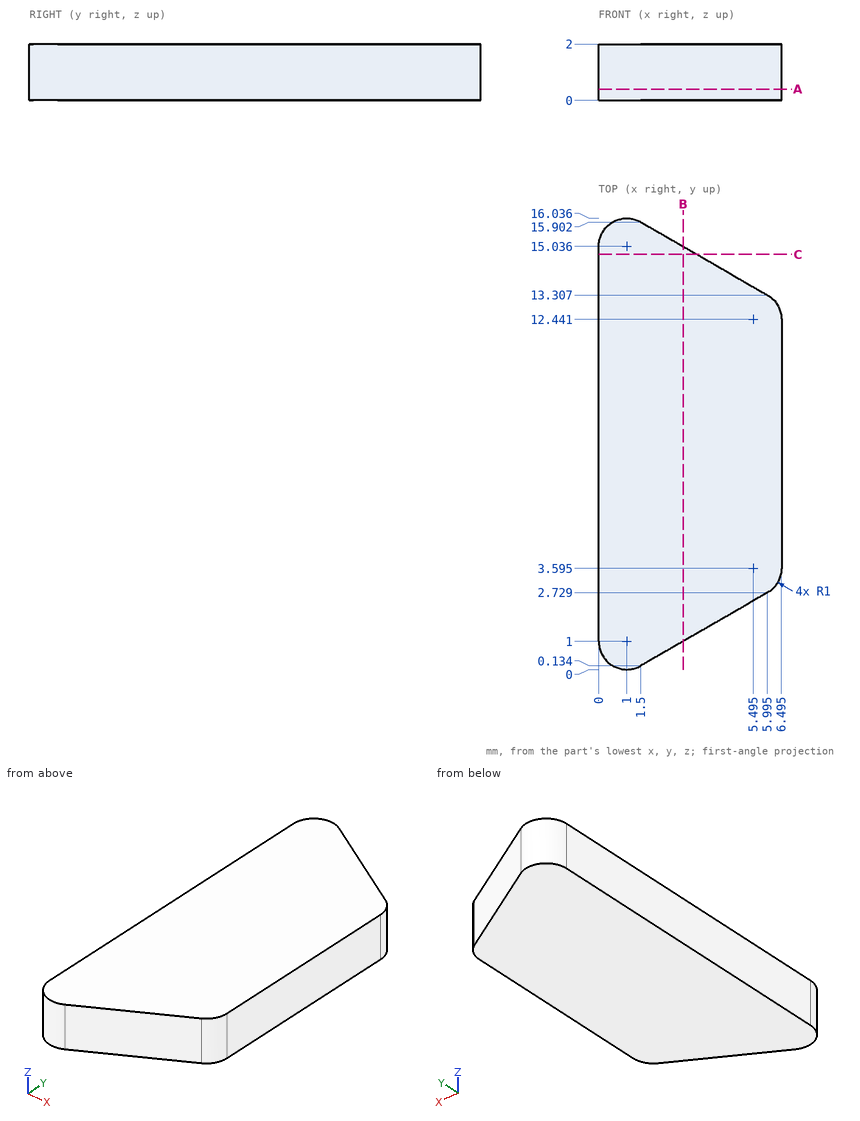
The drawing under review shows one solid part. Ordinate dimensions are in mm from its lowest x, y, z. Give positions to 0.01 mm unless a question says otherwise; leave off trailing zeros. Order: outer loops, then holes, each group sorted by start corner. A loop starts at its lowest first (then second) coordinate and runs counter-clockwise, first axis right, second up. Notation, with made-up numbers: (67.5, -23.5) - (126.5, -23.5) arc R21 cw to (126.5, -11.5) - close; hole circle Ø2 at (25, -7). An arc over 180 degrees is marked (long way). Answer as a JSON object with one key per item and string values. Group by question number.
Item 1: Take a section at C-C on y = 14.75. Give the boundary of the cut face in (x, z) (1 decimal).
Item 2: Clearance check with a flat-ended pin moving along its axis: pin 1 Ø1.5 at (x, y) = (1, 5.5) entering from -Z. State where the tip first meets the part, or that it passes through.
Item 3: Wall thickness on line 1 along Y through (x, z) = (6.25, 0.35) (1 decimal); line 2 along Y through (x, z) = (6, 0.3) (1 decimal); line 3 along X through (y, z) = (2.5, 1) (1 decimal): over which ranges is each line inside the solid? List them lowest first.
Item 4: Take a section at A-A on z = 0.4. Give the boundary of the cut face in (x, y) (1 decimal).
Item 5: Take a section at B-B on x = 3. Give the boundary of the cut face in (y, z).
Reported:
{
 "1": {"outline": "(0, 0) - (3.5, 0) - (3.5, 2) - (0, 2) - close"},
 "2": {"pin 1": "z = 0"},
 "3": {"line 1": "2.9 to 13.1", "line 2": "2.7 to 13.3", "line 3": "0 to 5.6"},
 "4": {"outline": "(0, 1) arc R1 ccw to (1.5, 0.1) - (6, 2.7) arc R1 ccw to (6.5, 3.6) - (6.5, 12.4) arc R1 ccw to (6, 13.3) - (1.5, 15.9) arc R1 ccw to (0, 15) - close"},
 "5": {"outline": "(1, 0) - (15.04, 0) - (15.04, 2) - (1, 2) - close"}
}
